Geometry: final body of the model. Coordinates: model frame, mm. Face numbers are marked on the shaded views. A direction names the side the tool comes from. Round coordinates to 2 decimals unless told otherwise and drop trailing zeros. Loops run counter-clockwise (first coordinate to the right, second up) from the corner with the lowest first, then second, coordinate; pieces in that order, holes last. Notation, with made-up numbers: (50, 26) - (92, 26) arc R6 ccw to (92, 36) - close; hole circle Ø6 at (84, -14). An arc over 180 degrees is marked (long way). Answer in a Markdown table with one row per item. Add a question column.
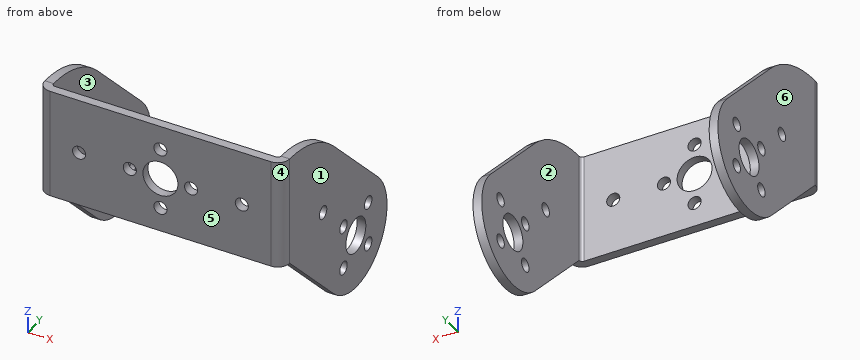
from build123d import *

# Parameters (mm, degrees)
SM_BASE_FLANGE_1_DEPTH   = 46.34
CUT_EXTRUDE_1_DEPTH      = 83.488760446
EXTRUDE_1_DEPTH          = 2
CUT_EXTRUDE_2_DEPTH      = 82.508925285
CUT_EXTRUDE_2_DEPTH_BACK = 82.508925285
SKETCH_9_R               = 4
SKETCH_9_R_2             = 1.5
SKETCH_10_R              = 4
SKETCH_10_R_2            = 1.5
CUT_EXTRUDE_3_DEPTH      = 2


# Sheet-metal steps are written as plain solids
with BuildPart() as part:
    # Sketch 1 → 基体-法兰1 (new body)
    with BuildSketch(Plane.XY):
        with BuildLine():
            Line((0, 39), (0, 0.7366))
            ThreePointArc((0, 0.7366), (0.215745145, 0.215745145), (0.7366, 0))
            Line((0.7366, 0), (51.2634, 0))
            ThreePointArc((51.2634, 0), (51.784254855, 0.215745145), (52, 0.7366))
            Line((52, 0.7366), (52, 39))
            Line((52, 39), (54, 39))
            Line((54, 39), (54, 0.7366))
            ThreePointArc((54, 0.7366), (53.198468417, -1.198468417), (51.2634, -2))
            Line((51.2634, -2), (0.7366, -2))
            ThreePointArc((0.7366, -2), (-1.198468417, -1.198468417), (-2, 0.7366))
            Line((-2, 0.7366), (-2, 39))
            Line((-2, 39), (0, 39))
        make_face()
    extrude(amount=SM_BASE_FLANGE_1_DEPTH)

    # 草图7 → 切除-拉伸1 (cut, through all)
    with BuildSketch(Plane.ZY.offset(2)):
        with BuildLine():
            ThreePointArc((46.34, 0.7366), (44.436988313, 10.303685809), (39.01766953, 18.41426953))
            Line((39.01766953, 18.41426953), (21.34, 36.091939059))
            Line((21.34, 36.091939059), (3.66233047, 18.41426953))
            Line((3.66233047, 18.41426953), (21.34, 0.7366))
            Line((21.34, 0.7366), (21.34, -3.161495831))
            Line((21.34, -3.161495831), (-1.543022836, -3.161495831))
            Line((-1.543022836, -3.161495831), (-1.543022836, 48.54205915))
            Line((-1.543022836, 48.54205915), (49.658153452, 48.54205915))
            Line((49.658153452, 48.54205915), (49.658153452, 0.7366))
            Line((49.658153452, 0.7366), (46.34, 0.7366))
        make_face()
    extrude(amount=-CUT_EXTRUDE_1_DEPTH, mode=Mode.SUBTRACT)

    # 草图8 → 凸台-拉伸1 (add)
    with BuildSketch(Plane.ZY.offset(2)):
        with BuildLine():
            Line((21.34, 36.091939059), (3.66233047, 18.41426953))
            ThreePointArc((3.66233047, 18.41426953), (3.66233047, 36.091939059), (21.34, 36.091939059))
        make_face()
    extrude_1 = extrude(amount=-EXTRUDE_1_DEPTH)

    # 镜向1: 凸台-拉伸1 across plane
    add(extrude_1.mirror(Plane(origin=(26, 0, 0), x_dir=(0, 0, 1), z_dir=(1, 0, 0))))

    # 草图9 → 切除-拉伸2 (cut, two sides: drawn at the far end of the back side and taken through both)
    with BuildSketch(Plane.ZY.offset(-52).offset(-CUT_EXTRUDE_2_DEPTH_BACK)):
        with Locations((12.501165235, 27.253104294)):
            Circle(SKETCH_9_R)
        with Locations((25.653351365, 14.100918164)):
            Circle(SKETCH_9_R_2)
        with Locations((7.551417767, 32.202851763)):
            Circle(SKETCH_9_R_2)
        with Locations((17.450912703, 32.202851763)):
            Circle(SKETCH_9_R_2)
        with Locations((17.450912703, 22.303356826)):
            Circle(SKETCH_9_R_2)
        with Locations((7.551417767, 22.303356826)):
            Circle(SKETCH_9_R_2)
    extrude(amount=CUT_EXTRUDE_2_DEPTH + CUT_EXTRUDE_2_DEPTH_BACK, mode=Mode.SUBTRACT)

    # 草图10 → 切除-拉伸3 (cut)
    with BuildSketch(Plane(origin=(0, 0, 0), x_dir=(1, 0, 0), z_dir=(0, 1, 0))):
        with Locations(Location((26, -33.84, 0), (0, 0, 270))):
            Circle(SKETCH_10_R)
        with Locations(Location((26, -26.84, 0), (0, 0, 270))):
            Circle(SKETCH_10_R_2)
        with Locations(Location((33, -33.84, 0), (0, 0, 270))):
            Circle(SKETCH_10_R_2)
        with Locations(Location((26, -40.84, 0), (0, 0, 270))):
            Circle(SKETCH_10_R_2)
        with Locations(Location((19, -33.84, 0), (0, 0, 270))):
            Circle(SKETCH_10_R_2)
        with Locations(Location((7.4, -33.84, 0), (0, 0, 270))):
            Circle(SKETCH_10_R_2)
        with Locations(Location((44.6, -33.84, 0), (0, 0, 270))):
            Circle(SKETCH_10_R_2)
    extrude(amount=-CUT_EXTRUDE_3_DEPTH, mode=Mode.SUBTRACT)


solid = part.part
1) Contact query for flat-ended pins moving along their axis: pin 1 Ø3 at (x, y) = (18, -1) entering from -Z; pin 2 Ø10 at (x, z) = (42, 33) entering from +Y. Output: stop coordinate, or through.
2) Section A-A, the plane x = 44.6. Return the cut outline in (y, z).
3) Reachability of the marked faces 1 and 2 from +Z, -Z, +X, -X, +Y, -Y: full face, straight path, thin tool, end or side. Return the list, or none.
4) Section D-D, the plane x = 26. Return the cut outline in (y, z).
5) Section B-B, the plane z = 7.5. Return the cut outline in (x, y), and give its area (3 significant figures).
6) Section C-C, the plane y = 11. Return the cut outline in (x, z), and give its area (3 significant figures).
7) Pull-direction query (X, two-part tool) for the marked faces 3, 4, 5 and 6; classes: pulls with the +X half, pulls with the -X half, needs draft (parallel to the pull), parting line crosses it, or undercut.
8) Material intervals for line 1 along X through (y, z) = (26, 8.5); line 2 along X through (y, z) = (-0.75, 33.84); line 3 along Y through (x, z) = (44.5, 28.5), sorted ascending. Write a range as from..to.
Evaluation:
| question | item | result |
|---|---|---|
| 1 | pin 1 | stops at z = 21.34 |
| 1 | pin 2 | stops at y = 0 |
| 2 | outline | (-2, 21.34) - (0, 21.34) - (0, 32.34) - (-2, 32.34) - close; (-2, 35.34) - (0, 35.34) - (0, 46.34) - (-2, 46.34) - close |
| 3 | face 1 | +Z, -Z, +X, +Y, -Y |
| 3 | face 2 | +Z, -Z, +Y |
| 4 | outline | (-2, 21.34) - (0, 21.34) - (0, 25.34) - (-2, 25.34) - close; (-2, 28.34) - (0, 28.34) - (0, 29.84) - (-2, 29.84) - close; (-2, 37.84) - (0, 37.84) - (0, 39.34) - (-2, 39.34) - close; (-2, 42.34) - (0, 42.34) - (0, 46.34) - (-2, 46.34) - close |
| 5 | outline | (-2, 14.58) - (0, 14.58) - (0, 20.8) - (-2, 20.8) - close; (-2, 23.8) - (0, 23.8) - (0, 30.7) - (-2, 30.7) - close; (-2, 33.7) - (0, 33.7) - (0, 38.71) - (-2, 38.71) - close; (52, 14.58) - (54, 14.58) - (54, 20.8) - (52, 20.8) - close; (52, 23.8) - (54, 23.8) - (54, 30.7) - (52, 30.7) - close; (52, 33.7) - (54, 33.7) - (54, 38.71) - (52, 38.71) - close |
| 5 | area | 72.5 mm² |
| 6 | outline | (-2, 11.08) - (0, 11.08) - (0, 44.14) - (-2, 44.14) - close; (52, 11.08) - (54, 11.08) - (54, 44.14) - (52, 44.14) - close |
| 6 | area | 132 mm² |
| 7 | face 3 | undercut |
| 7 | face 4 | pulls with the +X half |
| 7 | face 5 | needs draft |
| 7 | face 6 | pulls with the -X half |
| 8 | line 1 | x = -2..0, 52..54 |
| 8 | line 2 | x = -1.56..5.9, 8.9..17.5, 20.5..22, 30..31.5, 34.5..43.1, 46.1..53.56 |
| 8 | line 3 | y = -2..0 |
